Autodesk Inventor part; units mm, degrees
ref_plane "YZ Plane" through (0, 0, 0) normal (1, 0, 0) x (0, 1, 0)
ref_plane "XZ Plane" through (0, 0, 0) normal (0, 1, 0) x (-1, 0, 0)
ref_plane "XY Plane" through (0, 0, 0) normal (0, 0, 1) x (1, 0, 0)
sketch "Sketch1" plane through (0, 0, 0) normal (0, 0, 1) x (1, 0, 0)
  circle A0 centre (0, 0) radius 12.5
  dimension "d0" = 25
extrude "Extrusion1" add sketch "Sketch1" along normal blind 60
sketch "Sketch14" plane through (0, 0, 0) normal (0, 0, -1) x (-1, 0, 0)
  line L0 (0, 0) -> (0, 1.5)
  circle A0 centre (0, 0) radius 12.5
  line L1 (0, 1.5) -> (-12.4097, 1.5)
  line L2 (0, 0) -> (-1.8933, 0)
  line L3 (0, 1.5) -> (12.4097, 1.5)
  line L4 (0, -1.5) -> (-12.4097, -1.5)
  line L5 (0, -1.5) -> (12.4097, -1.5)
  dimension "d71" = 1.5
extrude "Extrusion10" add sketch "Sketch14" along normal blind 40 contours A0 L5 L4 L1 L3
sketch "Sketch16" plane through (0, 0, 60) normal (0, 0, 1) x (1, 0, 0)
  arc A0 (-12.4097, -1.5) -> (12.4097, -1.5) centre (0, 0) ccw
  line L0 (-10, -7.5) -> (10, -7.5)
  line L1 (12.4097, -1.5) -> (-12.4097, -1.5)
  dimension "d83" = 20
extrude "Extrusion12" cut sketch "Sketch16" against normal blind 10 contours L0 A0
sketch "Sketch17" plane through (0, 0, 0) normal (0, 0, -1) x (-1, 0, 0)
  line L0 (-12.4097, 1.5) -> (12.4097, 1.5)
  arc A0 (12.4097, 1.5) -> (-12.4097, 1.5) centre (0, 0) ccw
extrude "Extrusion13" add sketch "Sketch17" along normal up to surface (40 mm away)
sketch "Sketch15" plane through (-12.4097, 1.5, 0) normal (0, 1, 0) x (1, 0, 0)
  line L0 (0, 0) -> (0, 40)
  line L1 (0, 40) -> (24.8193, 40)
  circle A0 centre (12.4097, 35) radius 1.5
  circle A1 centre (12.4097, 8) radius 1.5
  point P0 (12.4097, 0)
  dimension "d79" = 3
  dimension "d80" = 5
  dimension "d81" = 3
  dimension "d82" = 27
extrude "Extrusion11" cut sketch "Sketch15" along normal mid plane 22
sketch "Sketch18" plane through (-10, -7.5, 60) normal (0, -1, 0) x (1, 0, 0)
  arc A0 (6.5, -7) -> (3.5, -7) centre (5, -5) ccw
  arc A1 (16.5, -7) -> (13.5, -7) centre (15, -5) ccw
  circle A2 centre (5, -5) radius 2.5
  circle A3 centre (15, -5) radius 2.5
  point P0 (10, -60)
  point P1 (13.5, -7)
  point P2 (16.5, -7)
  point P3 (3.5, -7)
  point P4 (6.5, -7)
extrude "Extrusion14" cut sketch "Sketch18" against normal blind 22
sketch "Sketch19" plane through (0, 0, -40) normal (0, 0, -1) x (-1, 0, 0)
  arc A0 (12.4097, -1.5) -> (-12.4097, -1.5) centre (0, 0) ccw
  line L0 (7.5, 10) -> (-7.5, 10)
  dimension "d90" = 15
extrude "Extrusion15" cut sketch "Sketch19" against normal blind 40
sketch "Sketch20" plane through (0, 0, 60) normal (0, 0, 1) x (1, 0, 0)
  arc A0 (10, -7.5) -> (-10, -7.5) centre (0, 0) ccw
  line L0 (-7.5, 10) -> (7.5, 10)
  dimension "d93" = 15
extrude "Extrusion16" cut sketch "Sketch20" against normal blind 12
properties part number "link2"
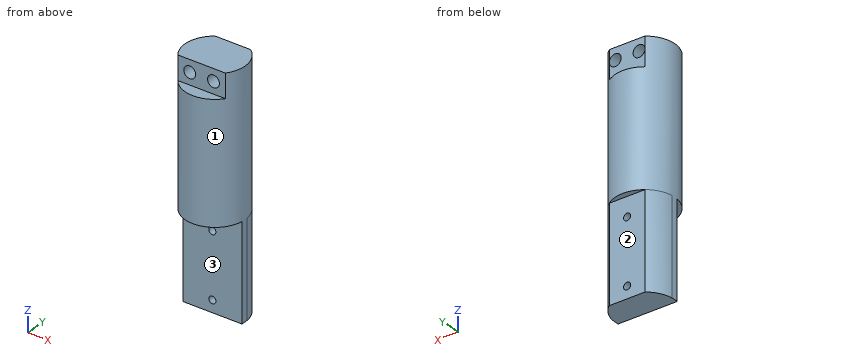
Geometry check sheet. Reference: the model listing, model coordinates, mm. Face numbers are marked on the shaded views. A direction names the side the tool comes from. Coordinates: 2 decimals unless noted, no trailing zeros. Order: outer loops, then holes, each group sorted by start corner. A loop starts at its lowest first (then second) coordinate and runs counter-clockwise, first axis right, second up.
Item 1: Section check B-B (z = -35). Enter the section's corners in (x, y), plus the area to 3 significant figures.
Item 2: Section check C-C (x = 5). Enter the section's corners in (y, z), plus the area to 3 significant figures.
Item 3: Section check A-A (y = 7.75). Enter the section's corners in (x, z), plus the area to 3 significant figures.
Item 4: Section check D-D (x = -6.5). Enter the section's corners in (y, z).
Item 5: Tool access check on the marked faces 1, 2 and 3. Record the directions out of +Z, -Z, +X, -X, +Y, -Y that give a thin tool (end or side, any length) a straight path to the whole face; none if there is none.
Item 6: Scan lines: line 1 along Z through (x, y) = (-5, 3.25); line 2 along Z through (x, y) = (0, 1.5); line 3 along X through (y, z) = (-0.75, 55). Record each from-to range of solid material in increasing order.
Item 7: Depth check by flat-ended pin: pin 1 (5.5 mm diameter, centred on x = 3, y = -9, fed in from +Z); pin 2 (12.5 mm diameter, centred on x = 2.5, z = -29, fed in from -Y); pin 3 (2 mm diameter, centred on y = 2, z = 35.5, fed in from -X); pin 4 (3 mm diameter, centred on x = 2, z = 57, fed in from -Y). Enter the tip coordinate at first touch or a pass-through.
Check sheet entries:
1. outline: (-12.41, -1.5) - (-1.5, -1.5) - (-1.5, 10) - (-7.5, 10) arc R12.5 ccw to start; (1.5, -1.5) - (12.41, -1.5) arc R12.5 ccw to (7.5, 10) - (1.5, 10) - close
1. area: 223 mm2
2. outline: (-11.46, 0) - (-1.5, 0) - (-1.5, -40) - (10, -40) - (10, 0) - (11.46, 0) - (11.46, 48) - (10, 48) - (10, 52.5) - (-7.5, 52.5) - (-7.5, 50) - (-11.46, 50) - close; (-7.5, 57.5) - (10, 57.5) - (10, 60) - (-7.5, 60) - close
2. area: 1,690 mm2
3. outline: (-9.81, -40) - (9.81, -40) - (9.81, 60) - (-9.81, 60) - close; hole circle Ø5 at (-5, 55); hole circle Ø3 at (0, -35); hole circle Ø3 at (0, -8); hole circle Ø5 at (5, 55)
3. area: 1,910 mm2
4. outline: (-10.68, 0) - (-1.5, 0) - (-1.5, -40) - (10, -40) - (10, 0) - (10.68, 0) - (10.68, 48) - (10, 48) - (10, 53) - (-7.5, 53) - (-7.5, 50) - (-10.68, 50) - close; (-7.5, 57) - (10, 57) - (10, 60) - (-7.5, 60) - close
5. face 1: +Z, -Z
5. face 2: -Z, +X, -X, +Y
5. face 3: -Z, +X, -X, -Y
6. line 1: z = -40 to 52.5, 57.5 to 60
6. line 2: z = -40 to -36.5, -33.5 to -9.5, -6.5 to 60
6. line 3: x = -12.48 to -7.5, -2.5 to 2.5, 7.5 to 12.48
7. pin 1: stops at z = 60
7. pin 2: stops at y = -1.5
7. pin 3: stops at x = -12.46
7. pin 4: stops at y = -7.5
